from build123d import *


with BuildPart() as f2:
    # F2: sweep along a path in F0
    with BuildLine(Plane.XY) as f2_path:
        Line((0, 0), (0, -250))
        Line((0, -250), (150, -250))
        Line((150, -250), (150, 0))
    # F1 (on Front) → F2 (sweep)
    with BuildSketch(Plane.XZ):
        Polygon((1.1390872965, 2.75), (-1.1390872965, 2.75), (-2.75, 1.1390872965), (-2.75, -1.1390872965), (-1.1390872965, -2.75), (1.1390872965, -2.75), (2.75, -1.1390872965), (2.75, 1.1390872965), align=None)
    sweep(path=f2_path.line, transition=Transition.RIGHT)


solid = f2.part
Check sheet for the modelled part. Datum: model origin and axes. Units: mm. Give positions to 0.01 mm unless a question says otherwise; leave off trailing zeros. Order: outer loops, then holes, each group sorted by start corner. A loop starts at its lowest first (then second) coordinate and runs counter-clockwise, first axis right, second up. Notation, with made-up numbers: M -17.75,28.5 L 31.25,28.5 A17 cw 31.25,50.5 Z; hole C -25.5,39 d1. An arc over 180 degrees is marked long. Answer as CSV lines item,"result". Start each with the question number.
Item 1: Thickness scan on line 1 (X direction, y = -121, z = -0.15); line 2 (Y direction, x = 101.5, z = 0.5); line 3 (X direction, y = -197.5, z = 1.75). Record the ranges inside material, lowest first. Write a range as [from, to].
Item 2: Gauge pin test, flat end, axial feed: P1, Ø2, axis at x = 43, z = -2, coming from the +Y side. Record the tip position at first contact, or that the pin passes through.
Item 3: Cross-section at B-B on x = 74. Enter the section's corners in (y, z), plus the area to 3 significant figures.
Item 4: Cross-section at A-A on y = -213. Enter the section's corners in (x, z).
Established:
1,line 1,"x = [-2.75, 2.75], [147.25, 152.75]"
1,line 2,"y = [-252.75, -247.25]"
1,line 3,"x = [-2.14, 2.14], [147.86, 152.14]"
2,P1,"stops at y = -247.25"
3,outline,"M -252.75,-1.14 L -251.14,-2.75 L -248.86,-2.75 L -247.25,-1.14 L -247.25,1.14 L -248.86,2.75 L -251.14,2.75 L -252.75,1.14 Z"
3,area,"25.1 mm^2"
4,outline,"M -2.75,-1.14 L -1.14,-2.75 L 1.14,-2.75 L 2.75,-1.14 L 2.75,1.14 L 1.14,2.75 L -1.14,2.75 L -2.75,1.14 Z; M 147.25,-1.14 L 148.86,-2.75 L 151.14,-2.75 L 152.75,-1.14 L 152.75,1.14 L 151.14,2.75 L 148.86,2.75 L 147.25,1.14 Z"
